The figure shows three views and two pictorial views of one solid part (mm, origin at its lowest corner). Answer the questions. A direction names the side the tool comes from. Coordinates: 2 decimals unless noted, no trailing zeros. Order: outer loops, then holes, each group sorted by start corner. A loop starts at its lowest first (then second) coordinate and runs counter-clockwise, first axis right, second up. Notation, with made-up numbers: (67.25, -38.75) -> (83.25, -38.75) arc R10 cw to (83.25, -25.75) -> close; hole circle Ø1 at (64, -39). An arc over 180 degrees is marked (long way). Use one line per item in the form item = value.
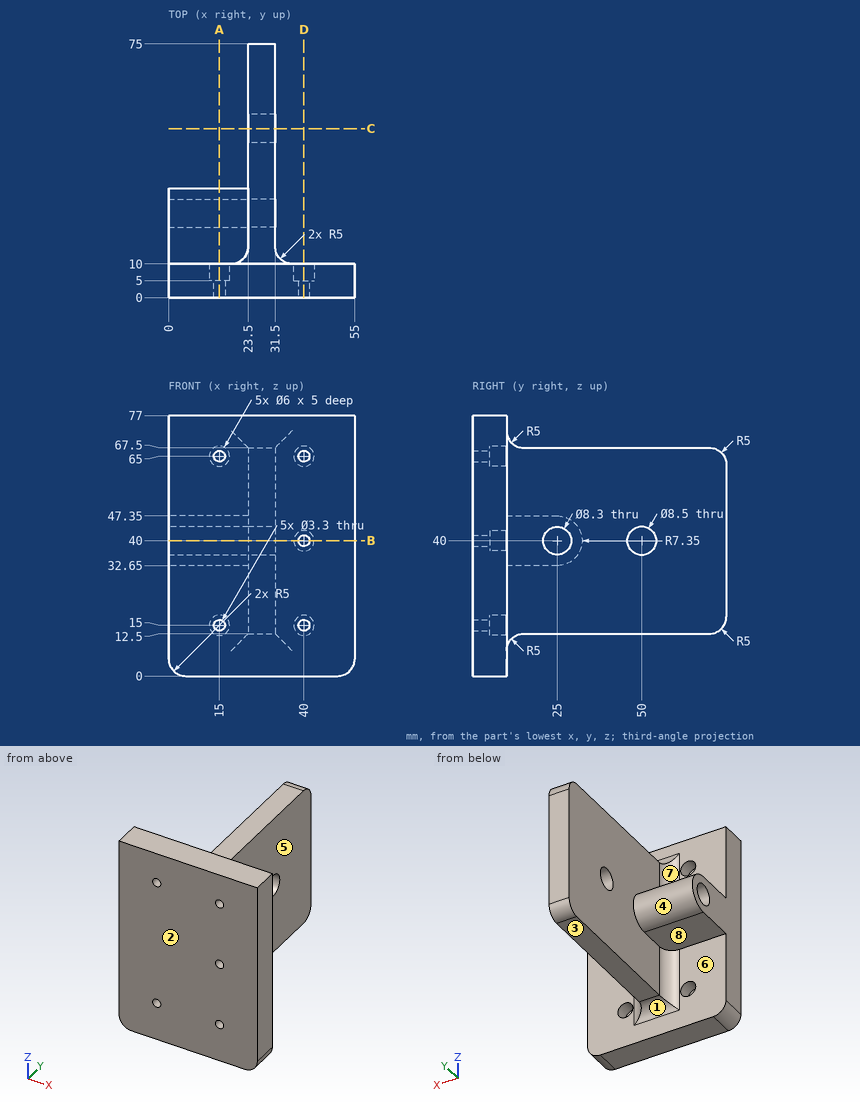
(1) Each of these flat-tipped pins is pushed along its axis until it touches: P1, Ø4, axis at y = 57.5, z = 67, coming from the -X side; P2, Ø4, axis at x = 28, y = 56, coming from the +Z side; P3, Ø3, axis at x = 40, z = 15, coming from the -Y side; P4, Ø3, axis at y = 27, z = 66.5, coming from the +X side. Where does it stop, or does it pass through?
Data:
P1 = 23.5
P2 = 67.5
P3 = through
P4 = 31.5
(2) Section C-C on y = 50 is taken. Write down the section's boundary in (x, z), plus the area to 3 significant figures.
Data:
outline = (23.5, 12.5) -> (31.5, 12.5) -> (31.5, 35.75) -> (23.5, 35.75) -> close; (23.5, 44.25) -> (31.5, 44.25) -> (31.5, 67.5) -> (23.5, 67.5) -> close
area = 372 mm²
(3) The mould has two halves that part along Y. Classify the marked faces 1, 2 and 3: released by +Y, released by -Y, zero draft, split by the parting line, or undercut.
Data:
face_1 = released by +Y
face_2 = released by -Y
face_3 = zero draft
(4) Section A-A on x = 15 is taken. Write down the section's boundary in (y, z), plus the area to 3 significant figures.
Data:
outline = (0, 0) -> (10, 0) -> (10, 12) -> (5, 12) -> (5, 13.35) -> (0, 13.35) -> close; (0, 16.65) -> (5, 16.65) -> (5, 18) -> (10, 18) -> (10, 32.65) -> (25, 32.65) arc R7.35 ccw to (25, 47.35) -> (10, 47.35) -> (10, 62) -> (5, 62) -> (5, 63.35) -> (0, 63.35) -> close; (0, 66.65) -> (5, 66.65) -> (5, 68) -> (10, 68) -> (10, 77) -> (0, 77) -> close; hole circle Ø8.3 at (25, 40)
area = 928 mm²
(5) Section B-B on z = 40 is taken. Write down the section's boundary in (x, y), plus the area to 3 significant figures.
Data:
outline = (0, 0) -> (38.35, 0) -> (38.35, 5) -> (37, 5) -> (37, 10) -> (36.5, 10) arc R5 cw to (31.5, 15) -> (31.5, 20.85) -> (0, 20.85) -> close; (0, 29.15) -> (31.5, 29.15) -> (31.5, 45.75) -> (23.5, 45.75) -> (23.5, 32.35) -> (0, 32.35) -> close; (23.5, 54.25) -> (31.5, 54.25) -> (31.5, 75) -> (23.5, 75) -> close; (41.65, 0) -> (55, 0) -> (55, 10) -> (43, 10) -> (43, 5) -> (41.65, 5) -> close
area = 1,220 mm²
(6) Straight lines are drawn through the part: line 1 along X through (y, z) = (7.6, 15); line 2 along Z through (x, y) = (40, 3); line 3 along Y through (x, z) = (27, 40). For each, find the intervals that lie inside material, in ascending order.
Data:
line_1 = 0 to 12, 18 to 37, 43 to 55
line_2 = 0 to 13.35, 16.65 to 38.35, 41.65 to 63.35, 66.65 to 77
line_3 = 0 to 20.85, 29.15 to 45.75, 54.25 to 75
(7) Section D-D on x = 40 is taken. Write down the section's boundary in (y, z).
Data:
outline = (0, 0) -> (10, 0) -> (10, 12) -> (5, 12) -> (5, 13.35) -> (0, 13.35) -> close; (0, 16.65) -> (5, 16.65) -> (5, 18) -> (10, 18) -> (10, 37) -> (5, 37) -> (5, 38.35) -> (0, 38.35) -> close; (0, 41.65) -> (5, 41.65) -> (5, 43) -> (10, 43) -> (10, 62) -> (5, 62) -> (5, 63.35) -> (0, 63.35) -> close; (0, 66.65) -> (5, 66.65) -> (5, 68) -> (10, 68) -> (10, 77) -> (0, 77) -> close
(8) Which of the six approach directions +Z, -Z, +X, -X, +Y, -Y give full straight-line access (tool end or side, diameter ignored) to the marked faces 4, 5, 6, 7 and 8?
Data:
face_4 = -X, +Y
face_5 = +Z, -Z, +X, +Y
face_6 = +Y
face_7 = +Z, -X, +Y
face_8 = -Z, -X, +Y
